Input: part model. Units: mm. Frame: model coordinates. Coordinates: 2 decimals unless noted, no trailing zeros. Order: outer loops, then holes, each group sorted by start corner. A loop starts at its lowest first (then second) coordinate and runs counter-clockwise, first axis right, second up. Notation, with made-up numbers: (-2, -1.75) -> (38, -1.75) arc R24 cw to (38, 29.25) -> close; hole circle Ø7 at (70.5, 82.5). An arc over 180 degrees is marked (long way). Answer as CSV lines item,"result".
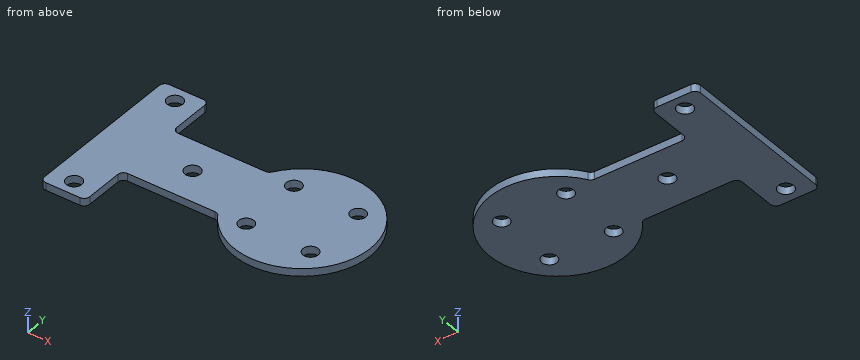
from build123d import *

# Parameters (mm, degrees)
SKETCH_1_R      = 2.05
SKETCH_1_R_2    = 2
EXTRUDE_1_DEPTH = 2
FILLET_1_R      = 1.5


with BuildPart() as part:
    # 草图1 → 凸台-拉伸1 (new body)
    with BuildSketch(Plane.XY):
        with BuildLine():
            Line((-42.723571429, -13.369911995), (-17.312028697, -13.369911995))
            ThreePointArc((-17.312028697, -13.369911995), (16.276428571, -4.369911995), (-17.312028697, 4.630088005))
            Line((-17.312028697, 4.630088005), (-42.723571429, 4.630088005))
            Line((-42.723571429, 4.630088005), (-42.723571429, 17.630088005))
            Line((-42.723571429, 17.630088005), (-54.723571429, 17.630088005))
            Line((-54.723571429, 17.630088005), (-54.723571429, -26.369911995))
            Line((-54.723571429, -26.369911995), (-42.723571429, -26.369911995))
            Line((-42.723571429, -26.369911995), (-42.723571429, -13.369911995))
        make_face()
        with Locations((-30.723571429, -4.369911995)):
            Circle(SKETCH_1_R, mode=Mode.SUBTRACT)
        with Locations((-48.723571429, 13.630088005)):
            Circle(SKETCH_1_R, mode=Mode.SUBTRACT)
        with Locations((-48.723571429, -22.369911995)):
            Circle(SKETCH_1_R, mode=Mode.SUBTRACT)
        with Locations((6.776428571, -12.869911995)):
            Circle(SKETCH_1_R_2, mode=Mode.SUBTRACT)
        with Locations((-10.223571429, -12.869911995)):
            Circle(SKETCH_1_R_2, mode=Mode.SUBTRACT)
        with Locations((-10.223571429, 4.130088005)):
            Circle(SKETCH_1_R_2, mode=Mode.SUBTRACT)
        with Locations((6.776428571, 4.130088005)):
            Circle(SKETCH_1_R_2, mode=Mode.SUBTRACT)
    extrude(amount=EXTRUDE_1_DEPTH)

    # 圆角1
    fillet_1_edges = [part.edges().sort_by_distance(p)[0] for p in [
        (-42.723571429, -13.369911995, 1),
        (-42.723571429, -26.369911995, 1),
        (-54.723571429, -26.369911995, 1),
        (-54.723571429, 17.630088005, 1),
        (-42.723571429, 17.630088005, 1),
        (-42.723571429, 4.630088005, 1),
        (-17.312028697, 4.630088005, 1),
        (-17.312028697, -13.369911995, 1),
    ]]
    fillet(fillet_1_edges, radius=FILLET_1_R)


solid = part.part
1. Cut plane D-D (x = -28). Return the cut outline in (y, z).
Findings:
outline,"(-13.37, 0) -> (4.63, 0) -> (4.63, 2) -> (-13.37, 2) -> close"
2. Cut plane B-B (x = 6.5). Return the cut outline in (y, z), plus the area to 3 significant figures.
Findings:
outline,"(-20.38, 0) -> (-14.85, 0) -> (-14.85, 2) -> (-20.38, 2) -> close; (-10.89, 0) -> (2.15, 0) -> (2.15, 2) -> (-10.89, 2) -> close; (6.11, 0) -> (11.64, 0) -> (11.64, 2) -> (6.11, 2) -> close"
area,"48.2 mm2"
3. Ray query, line 1 along X through (y, z) = (5.5, 1.75); line 2 along X through (y, z) = (-22.5, 1.6); line 3 along Y through (x, z) = (-47, 0.7). Return the intervals inside material, ascending.
Findings:
line 1,"x = -54.72 to -42.58, -16.78 to -11.68, -8.77 to 5.32, 8.23 to 13.33"
line 2,"x = -54.72 to -50.77, -46.68 to -42.72"
line 3,"y = -26.37 to -23.48, -21.26 to 12.52, 14.74 to 17.63"
4. Cut plane A-A (y = -5.5). Return the cut outline in (x, z), plus the area to 3 significant figures.
Findings:
outline,"(-54.72, 0) -> (-32.43, 0) -> (-32.43, 2) -> (-54.72, 2) -> close; (-29.01, 0) -> (16.24, 0) -> (16.24, 2) -> (-29.01, 2) -> close"
area,"135 mm2"
5. Contact query for flat-ended pins moving along their axis: pin 1 (1 mm diameter, centred on y = -20.5, z = 1, fed in from +X); pin 2 (1 mm diameter, centred on x = -39.5, z = 1, fed in from +Y). Output: stop coordinate, or through.
Findings:
pin 1,"stops at x = 7.2"
pin 2,"stops at y = 4.63"
6. Cut plane C-C (z = 0.6). Return the cut outline in (x, y).
Findings:
outline,"(-54.72, -24.87) arc R1.5 ccw to (-53.22, -26.37) -> (-44.22, -26.37) arc R1.5 ccw to (-42.72, -24.87) -> (-42.72, -14.87) arc R1.5 cw to (-41.22, -13.37) -> (-18.16, -13.37) arc R1.5 cw to (-16.89, -14.06) arc R18 ccw (long way) to (-16.89, 5.32) arc R1.5 cw to (-18.16, 4.63) -> (-41.22, 4.63) arc R1.5 cw to (-42.72, 6.13) -> (-42.72, 16.13) arc R1.5 ccw to (-44.22, 17.63) -> (-53.22, 17.63) arc R1.5 ccw to (-54.72, 16.13) -> close; hole circle Ø4.1 at (-48.72, -22.37); hole circle Ø4.1 at (-48.72, 13.63); hole circle Ø4.1 at (-30.72, -4.37); hole circle Ø4 at (-10.22, -12.87); hole circle Ø4 at (-10.22, 4.13); hole circle Ø4 at (6.78, -12.87); hole circle Ø4 at (6.78, 4.13)"
